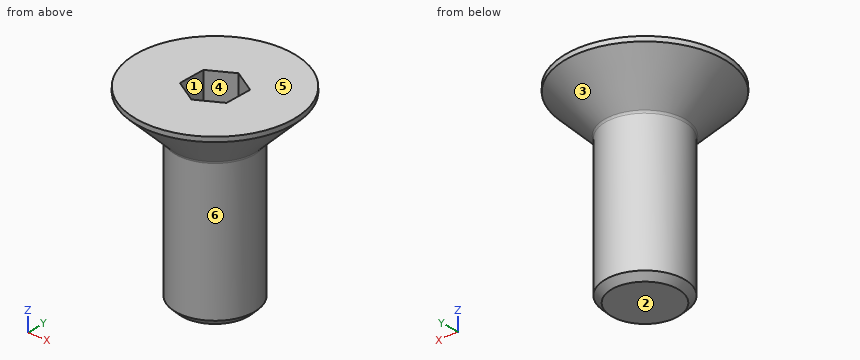
Autodesk Inventor part; units mm, degrees
ref_plane "MSC_PF1" through (0, 0, 0) normal (1, 0, 0) x (0, 1, 0)
ref_plane "MSC_PT1" through (0, 0, 0) normal (0, 0, -1) x (-1, 0, 0)
ref_plane "YZ Plane" through (0, 0, 0) normal (1, 0, 0) x (0, 1, 0)
sketch "Sketch1" plane through (0, 0, 0) normal (0, 1, 0) x (-1, 0, 0)
  point P0 (0, 0)
sketch "Sketch2" plane through (0, 0, 0) normal (0, 1, 0) x (-1, 0, 0)
  line L0 (-2.5, -12) -> (0, -12)
  line L1 (-2.5, -2.8) -> (-2.5, -12)
  line L2 (-5, -0.3) -> (-2.5, -2.8)
  line L3 (-5, 0) -> (-5, -0.3)
  line L4 (0, 0) -> (-5, 0)
  line L5 (0, -12) -> (0, 0)
  line L6 (0, -12) -> (0, 0)
  line L7 (0, -14.4) -> (0, 2.4)
  line L8 (1, 0) -> (-6, 0)
  dimension "d3" = 5
  dimension "d5" = 2.5
  dimension "d7" = 12
  dimension "ParC" = 0.3
  dimension "d22" = 0
  dimension "d23" = 0
  dimension "d43" = 45
revolve "Revolution1" add sketch "Sketch2" angle 360 about axis through (0, 0, -12) along (0, 0, -1)
sketch "Sketch3" plane through (0, 0, 0) normal (0, 0, 1) x (1, 0, 0)
  line L0 (-1.5, 0.866) -> (-1.5, -0.866)
  line L1 (0, 1.7321) -> (-1.5, 0.866)
  line L2 (1.5, 0.866) -> (0, 1.7321)
  line L3 (1.5, -0.866) -> (1.5, 0.866)
  line L4 (0, -1.7321) -> (1.5, -0.866)
  line L5 (-1.5, -0.866) -> (0, -1.7321)
  circle A0 centre (0, 0) radius 1.5 construction
  circle A1 centre (0, 0) radius 2.5 construction
  dimension "d11" = 3
  dimension "d13" = 120
  dimension "d15" = 120
extrude "Extrusion1" cut sketch "Sketch3" against normal blind 2.3
fillet "Fillet1" radius 0.2 1 edges at (-2.5, 0, -2.8)
chamfer "Chamfer1" distance 0.4 angle 45 1 edges at (-2.5, 0, -12) measured on face at (-0.599, -2.4272, -8.9609)
thread "Thread1"
ref_plane "MSC_PF1" through (0, 0, 0) normal (1, 0, 0) x (0, 1, 0)
ref_plane "MSC_PT1" through (0, 0, 0) normal (0, 0, -1) x (-1, 0, 0)
equation "\"d3\" = 0.5 * dk"
equation "\"d5\" = 0.5 * NND"
equation "\"d7\" = NLG"
equation "\"d43\" = 0.5 * ang"
equation "\"d18\" = r"
equation "\"d19\" = 0.5 * PTC"
equation "\"d39\" = 0.5 * PTC"
equation "\"d11\" = ParS"
equation "\"d16\" = ParT"
equation "\"NND\" = 5"
equation "\"PTC\" = 0.8"
equation "\"ParK\" = 2.8"
equation "\"ParS\" = 3"
equation "\"ParT\" = 2.3"
equation "\"r\" = 0.2"
equation "\"NLG\" = 12"
equation "\"ang\" = 90deg"
equation "\"THREADDIA\" = NND"
properties part number "ISO 10642 - M5x12" material "Steel, Mild"
Build history of the part. All positions in model axes, mm. Face numbers are marked on the shaded views. A direction names the side the tool comes from. Give positions to 0.01 mm unless a question says otherwise; leave off trailing zeros. Order: outer loops, then holes, each group sorted by start corner. A loop starts at its lowest first (then second) coordinate and runs counter-clockwise, first axis right, second up. Notation, with made-up numbers: M -14,-39 L -6,-39 A31 cw -6,-5 Z; hole C 32,81.5 d7. An arc over 180 degrees is marked long. Put each result on its own line as item: value.
Item 1: Probe line 1 (Y direction, x = 2, z = -7.75); line 2 (Z direction, x = -1.25, y = 0). List the from-to ranges inside material, lowest first. Write a range as [from, to].
From the geometry:
line 1: y = [-1.5, 1.5]
line 2: z = [-12, -2.3]
Item 2: Two-plate mould, pull along Y, no slides. Class the marked faces 1, 2 and 3: +Y half, -Y half, draft (parallel to the pull), parting line (faces both ways), or undercut.
From the geometry:
face 1: undercut
face 2: draft
face 3: parting line
Item 3: Flat gauge pins, fed straight in: pin 1 Ø5 at (x, z) = (-2.5, -4.5) entering from +Y; pin 2 Ø1.5 at (x, y) = (-2, 3.5) entering from -Z; pin 3 Ø1.5 at (x, y) = (0.5, 0) entering from +Z. Where does each tip first touch, or does it go through?
From the geometry:
pin 1: stops at y = 2.7
pin 2: stops at z = -2.02
pin 3: stops at z = -2.3
Item 4: 3-axis set-ups, long thin cutter, end or side, ignore diameter. For the marked faces 4, 5 and 6: which of +Z, -Z, +X, -X, +Y, -Y reach the whole face in a straight line?
From the geometry:
face 4: +Z
face 5: +Z, +X, -X, +Y, -Y
face 6: -Z
Item 5: Slice it at A-A, the plane z = -8.75. Write the cut outline in (x, y).
From the geometry:
outline: C 0,0 d5
